Input: dimensioned drawing with shaded views. Units: mm. Origin: part minimum x, y, z. Give positions to 0.01 mm unless a question says otherwise; leave off trailing zeros. Order: outer loops, then holes, each group sorted by start corner. A loop starts at its lowest first (then second) coordinate and runs counter-clockwise, first axis right, second up.
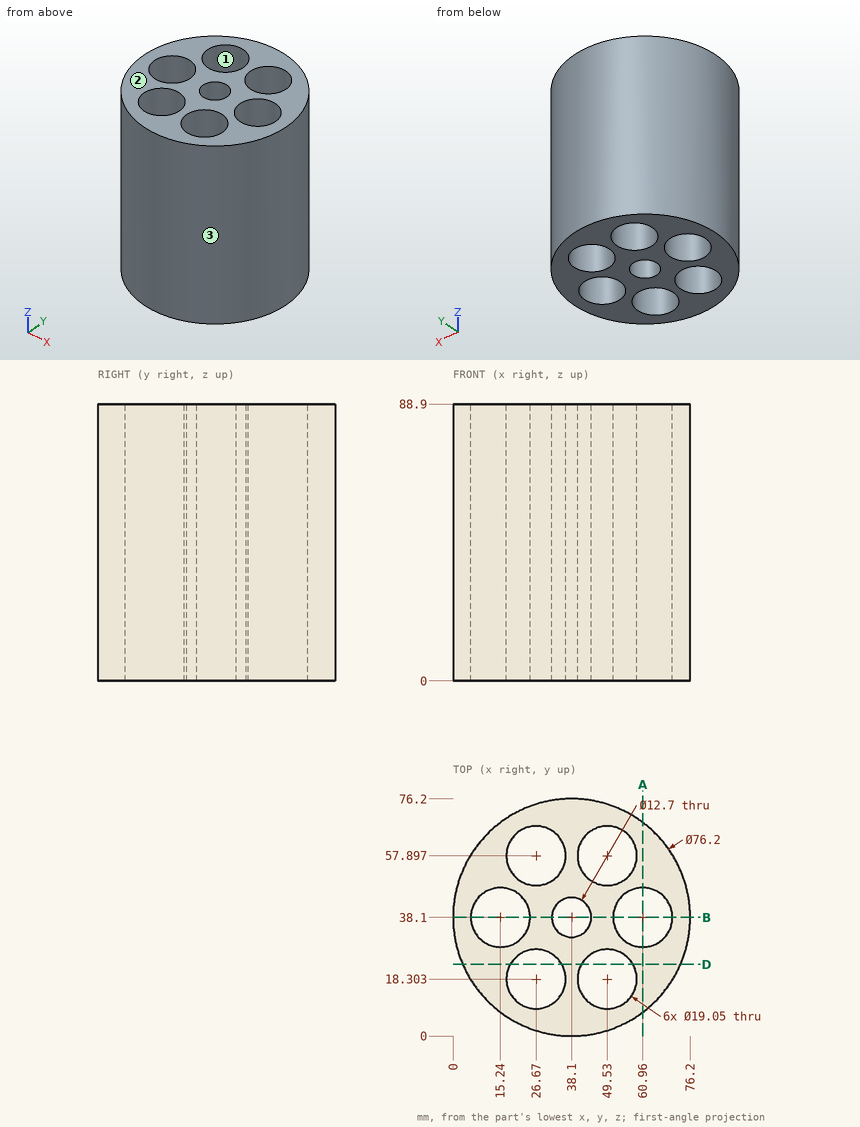
1) Line query: probe 1 along X at (y, z) = (38.5, 64.5); probe 2 along Y at (x, z) = (45, 78) (1 decimal); probe 3 along Y at (x, z) = (26, 63) (1 decimal). Output: solid intervals per line, ascending.
2) Cut plane D-D (y = 23). Return the cut outline in (x, z), then the cut area to 3 significant figures.
3) Cut plane B-B (y = 38.1). Count the separate pieces of the cut face and the enclosed holes in it, then the cut area to 3 significant figures.
4) First-contact query: P1, Ø22, axis at x = 26.67, y = 57.9, coming from the -Z side; P2, Ø15, axis at x = 60.96, y = 38.1, coming from the -Z side; P3, Ø10, axis at y = 63, z = 21, coming from the +X side; P4, Ø2, axis at y = 18, z = 10.5, coming from the -X side. Flat tips, straight axial feed; report the tip coordinate or a pass-through.
5) Pull-direction query (X, two-part tool) for the marked faces 1, 2 and 3; classes: pulls with the +X half, pulls with the -X half, needs draft (parallel to the pull), parting line crosses it, or undercut.
6) Cut plane A-A (x = 60.96). Return the cut outline in (y, z) (1 decimal), then the cut area to 3 significant figures.
Geometry says:
1. probe 1: x = 0 to 5.72, 24.76 to 31.76, 44.44 to 51.44, 70.48 to 76.2
1. probe 2: y = 0.6 to 9.9, 26.7 to 49.5, 66.3 to 75.6
1. probe 3: y = 2 to 8.8, 27.8 to 48.4, 67.4 to 74.2
2. outline: (3.12, 0) - (18.38, 0) - (18.38, 88.9) - (3.12, 88.9) - close; (34.96, 0) - (41.24, 0) - (41.24, 88.9) - (34.96, 88.9) - close; (57.82, 0) - (73.08, 0) - (73.08, 88.9) - (57.82, 88.9) - close
2. area: 3,270 mm2
3. separate pieces: 4
3. enclosed holes: 0
3. area: 2,260 mm2
4. P1: stops at z = 0
4. P2: passes through
4. P3: stops at x = 70.59
4. P4: stops at x = 5.13
5. face 1: undercut
5. face 2: needs draft
5. face 3: parting line crosses it
6. outline: (7.6, 0) - (28.6, 0) - (28.6, 88.9) - (7.6, 88.9) - close; (47.6, 0) - (68.6, 0) - (68.6, 88.9) - (47.6, 88.9) - close
6. area: 3,730 mm2
